Read the model definition and answer for the solid it produces. Units are mm, in the model's axes. A direction names the side the tool comes from. Round coordinates to 2 decimals unless told otherwise and drop trailing zeros. Loops run counter-clockwise (first coordinate to the right, second up) from the corner with the lowest first, then second, coordinate; pieces in that order, holes last. Notation, with made-up numbers: (27, 29) - (64, 29) arc R15 cw to (64, 55) - close; hole circle Ø2 at (23, 89.25). An arc over 180 degrees is marked (long way). Use CSV: the item, a comma, the result in double quotes. Start each with the question number.
1. Find section D-D (y = 176.5). Give the vertices of the cut face in (x, z) (3 decimals), and give its area (3 significant figures).
2. Find section B-B (x = 95). Give the vertices of the cut face in (y, z), and give its area (3 significant figures).
3. Find section A-A (y = 110). Give the vertices of the cut face in (x, z) (3 decimals).
4. A tool of negligible diameter and unlimited length cuts with its end or side. For faces 4 (the flat face through (45.812, 132, 3)), 5 (the flat face through (130, 195.493, 3)), 6 (the flat face through (134, 103, 3)), from which of +Z, -Z, +X, -X, +Y, -Y can it reach the whole face along a straight path? Write none if from no direction.
5. Find section C-C (y = 77). Give the vertices of the cut face in (x, z) (1 decimal), and give its area (4 significant figures).
6. Given pin 1 Ø3 at (y, z) = (199, 3.5) entering from +X; pin 2 Ø9.5 at (x, y) = (98.56, 178.59) entering from -Z; pin 3 Ø2 at (x, z) = (130.5, 2.5) entering from -Y; pin 4 Ø1.2 at (x, z) = (130.5, 2) entering from +Y, each flat-ended and moving along its own axis, determine where each tip first touches the part or whether it passes through.
7. Determine the mould class of faces 1 (the flat face through (6, 8, 3)), 2 (the flat face through (0, 103, 3)), 3 (the flat face through (81, 103, 0)) for opening direction X: +X half, -X half, draft (parallel to the pull), parting line (faces both ways), or undercut.
8. Consider line 1 along X through (y, z) = (79.5, 4.55) (1 decimal); line 2 along Y through (x, z) = (86, 1.3); line 3 along X through (y, z) = (18, 3.65) (3 decimals). Determine where each line is inside the solid, lowest interval first.
Autodesk Inventor part; units mm, degrees
ref_plane "YZ Plane" through (0, 0, 0) normal (1, 0, 0) x (0, 1, 0)
ref_plane "XZ Plane" through (0, 0, 0) normal (0, 1, 0) x (-1, 0, 0)
ref_plane "XY Plane" through (0, 0, 0) normal (0, 0, 1) x (1, 0, 0)
sketch "Sketch1" plane through (0, 0, 0) normal (0, 0, 1) x (1, 0, 0)
  line L0 (0, 0) -> (128, 0)
  line L1 (128, 0) -> (128, 203.5927)
  line L2 (128, 203.5927) -> (0, 203.5927)
  line L3 (0, 203.5927) -> (0, 0)
  line L4 (0, 0) -> (-77.2375, 168.1052) construction
  line L5 (-77.2375, 168.1052) -> (0, 203.5927) construction
  line L6 (2.875, 195.5927) -> (9.125, 195.5927)
  line L7 (9.125, 195.5927) -> (9.125, 8)
  line L8 (9.125, 8) -> (2.875, 8)
  line L9 (2.875, 8) -> (2.875, 195.5927)
  dimension "d0" = 128
  dimension "d1" = 85
  dimension "d2" = 185
  dimension "d3" = 6.25
  dimension "d4" = 2.875
  dimension "d5" = 8
  dimension "d6" = 8
extrude "Extrusion1" add sketch "Sketch1" along normal blind 6
sketch "Sketch2" plane through (0, 0, 6) normal (0, 0, 1) x (1, 0, 0)
  line L0 (0, 0) -> (128, 0)
  line L1 (128, 0) -> (128, 203.5927)
  line L2 (128, 203.5927) -> (0, 203.5927)
  line L3 (128, 195.4927) -> (134, 195.4927)
  line L4 (134, 195.4927) -> (134, 8.1)
  line L5 (134, 8.1) -> (128, 8.1)
  line L6 (128, 8.1) -> (128, 195.4927)
  dimension "d9" = 8.1
  dimension "d10" = 8.1
  dimension "d11" = 6
extrude "Extrusion2" add sketch "Sketch2" against normal blind 6
fillet "Fillet1" radius 2 6 edges at (134, 195.4927, 3) (128, 203.5927, 3) (0, 203.5927, 3) (128, 0, 3) (134, 8.1, 3) (0, 0, 3)
sketch "Sketch3" plane through (0, 0, 6) normal (0, 0, 1) x (1, 0, 0)
  line L0 (9.125, 195.5927) -> (9.125, 8)
  line L1 (2, 0) -> (126, 0)
  line L2 (128, 195.4927) -> (128, 201.5927)
  line L3 (126, 203.5927) -> (2, 203.5927)
  circle A0 centre (38.5625, 178.5927) radius 8
  circle A1 centre (68.5625, 178.5927) radius 8
  circle A2 centre (98.5625, 178.5927) radius 8
  line L4 (45.8125, 118.5618) -> (91.3125, 118.5618)
  line L5 (91.3125, 118.5618) -> (91.3125, 145.0618)
  line L6 (91.3125, 145.0618) -> (45.8125, 145.0618)
  line L7 (45.8125, 145.0618) -> (45.8125, 118.5618)
  line L8 (45.8125, 118.5618) -> (91.3125, 145.0618) construction
  line L9 (91.3125, 118.5618) -> (45.8125, 145.0618) construction
  line L10 (45.8125, 71.7809) -> (91.3125, 71.7809)
  line L11 (91.3125, 71.7809) -> (91.3125, 98.2809)
  line L12 (91.3125, 98.2809) -> (45.8125, 98.2809)
  line L13 (45.8125, 98.2809) -> (45.8125, 71.7809)
  line L14 (45.8125, 71.7809) -> (91.3125, 98.2809) construction
  line L15 (91.3125, 71.7809) -> (45.8125, 98.2809) construction
  line L16 (45.8125, 25) -> (91.3125, 25)
  line L17 (91.3125, 25) -> (91.3125, 51.5)
  line L18 (91.3125, 51.5) -> (45.8125, 51.5)
  line L19 (45.8125, 51.5) -> (45.8125, 25)
  line L20 (45.8125, 25) -> (91.3125, 51.5) construction
  line L21 (91.3125, 25) -> (45.8125, 51.5) construction
  line L22 (68.5625, 178.5927) -> (68.5625, 131.8118) construction
  line L23 (68.5625, 131.8118) -> (68.5625, 85.0309) construction
  line L24 (68.5625, 85.0309) -> (68.5625, 38.25) construction
  point P0 (0, 0)
  dimension "d15" = 16
  dimension "d16" = 26.5
  dimension "d17" = 45.5
  dimension "d18" = 118.875
  dimension "d19" = 59.4375
  dimension "d20" = 30
  dimension "d21" = 30
  dimension "d22" = 25
  dimension "d23" = 25
extrude "Extrusion3" cut sketch "Sketch3" against normal blind 10
equation "\"d19\" = 0.5 * d18"
equation "\"d21\" = d20"
properties part number "NewControlPanel"
Filled sheet:
1,outline,"(0, 0) - (2.875, 0) - (2.875, 6) - (0, 6) - close; (9.125, 0) - (30.841, 0) - (30.841, 6) - (9.125, 6) - close; (46.284, 0) - (60.841, 0) - (60.841, 6) - (46.284, 6) - close; (76.284, 0) - (90.841, 0) - (90.841, 6) - (76.284, 6) - close; (106.284, 0) - (134, 0) - (134, 6) - (106.284, 6) - close"
1,area,"489 mm²"
2,outline,"(0, 0) - (171.43, 0) - (171.43, 6) - (0, 6) - close; (185.76, 0) - (203.59, 0) - (203.59, 6) - (185.76, 6) - close"
2,area,"1,140 mm²"
3,outline,"(0, 0) - (2.875, 0) - (2.875, 6) - (0, 6) - close; (9.125, 0) - (134, 0) - (134, 6) - (9.125, 6) - close"
4,face 4,"+Z, -Z"
4,face 5,"+Z, -Z, +X, +Y"
4,face 6,"+Z, -Z, +X, +Y, -Y"
5,outline,"(0, 0) - (2.9, 0) - (2.9, 6) - (0, 6) - close; (9.1, 0) - (45.8, 0) - (45.8, 6) - (9.1, 6) - close; (91.3, 0) - (134, 0) - (134, 6) - (91.3, 6) - close"
5,area,"493.5 mm²"
6,pin 1,"stops at x = 128"
6,pin 2,"passes through"
6,pin 3,"stops at y = 8.1"
6,pin 4,"stops at y = 195.49"
7,face 1,"undercut"
7,face 2,"-X half"
7,face 3,"draft"
8,line 1,"x = 0 to 2.9, 9.1 to 45.8, 91.3 to 134"
8,line 2,"y = 0 to 25, 51.5 to 71.78, 98.28 to 118.56, 145.06 to 203.59"
8,line 3,"x = 0 to 2.875, 9.125 to 134"
